For this review, take the finished solid that the model builds, in its own axes (mm). A direction names the side the tool comes from. Coordinates: 2 decimals unless noted, no trailing zeros. Loops run counter-clockwise (first coordinate to the right, second up) from the corner with the lowest first, then second, coordinate; pieces in that order, holes last. Notation, with made-up numbers: M -25,-8 L -13,-8 A24 ccw -13,19 Z; hole C 72,-5 d1. An arc over 180 degrees is marked long. Use one line per item in the form item = value.
```python
from build123d import *

# Parameters (mm, degrees)
SKETCH1_W           = 51.225
SKETCH1_H           = 33.05
BOSS_EXTRUDE1_DEPTH = 6.35
SKETCH8_R           = 1.25
CUT_EXTRUDE4_DEPTH  = 15
FILLET3_R           = 5.08
SKETCH10_R          = 3.35
SKETCH10_R_2        = 11.05
CUT_EXTRUDE5_DEPTH  = 4.7625
CHAMFER1_SIZE       = 0.25


with BuildPart() as part:
    # Sketch1 → Boss-Extrude1 (new body)
    with BuildSketch(Plane.XY):
        with Locations((-7.6125, 2.525)):
            Rectangle(SKETCH1_W, SKETCH1_H)
    extrude(amount=-BOSS_EXTRUDE1_DEPTH)

    # Sketch8 → Cut-Extrude4 (cut)
    with BuildSketch(Plane(origin=(0, 19.05, 0), x_dir=(1, 0, 0), z_dir=(0, 1, 0))):
        with Locations(Location((-29.725, 3.175, 0), (0, 0, 270))):
            Circle(SKETCH8_R)
        with Locations(Location((-14, 3.175, 0), (0, 0, 270))):
            Circle(SKETCH8_R)
        with Locations(Location((14.5, 3.175, 0), (0, 0, 270))):
            Circle(SKETCH8_R)
    extrude(amount=-CUT_EXTRUDE4_DEPTH, mode=Mode.SUBTRACT)

    # Fillet3
    fillet3_edges = [part.edges().sort_by_distance(p)[0] for p in [
        (18, -14, -3.175),
        (-33.225, -14, -3.175),
    ]]
    fillet(fillet3_edges, radius=FILLET3_R)

    # Sketch10 → Cut-Extrude5 (cut)
    with BuildSketch(Plane(origin=(0, 0, -6.35), x_dir=(-1, 0, 0), z_dir=(0, 0, -1))):
        with Locations((22.225, 0)):
            Circle(SKETCH10_R)
        Circle(SKETCH10_R_2)
    extrude(amount=-CUT_EXTRUDE5_DEPTH, mode=Mode.SUBTRACT)

    # Chamfer1
    chamfer1_edges = [part.edges().sort_by_distance(p)[0] for p in [
        (-29.725, 19.05, -4.425),
        (-14, 19.05, -4.425),
        (14.5, 19.05, -4.425),
    ]]
    chamfer(chamfer1_edges, length=CHAMFER1_SIZE)


solid = part.part
```
1. Tool access review of faces 1 (the face through (-31.78, -12.47, -3.22)), 2 (the face through (-28.486, 11.528, -3.338)), 3 (the face through (-22, 0, -1.587)): name each direction out of +Z, -Z, +X, -X, +Y, -Y from which nothing blocks a thin tool from reaching the whole face with its end or side.
Computed values:
face_1 = +Z, -Z, -X, -Y
face_2 = +Y
face_3 = -Z
2. Consider section D-D on z = -2.5. State how many separate pieces and enclosed holes the cut face has, plus the area to 3 significant figures.
Computed values:
separate_pieces = 1
enclosed_holes = 2
area = 1,170 mm2
3. Draft analysis for pull direction Z (two halves, no side actions). For faces 4 (the face through (2.395, -10.787, -4.002)), 5 (the face through (-14, 4.05, -3)), 6 (the face through (-8, 3, 0)), state which applies: +Z half, -Z half, draft (parallel to the pull), parting line (faces both ways), or undercut.
Computed values:
face_4 = draft
face_5 = undercut
face_6 = +Z half
4. Wall thickness on line 1 along Y through (x, z) = (0, -4.95); line 2 along X through (y, z) = (14, -3.5) (3 decimals); line 3 along X through (y, z) = (-6, -5.5) (3 decimals): over which ranges is each line inside the solid? List them lowest first. Write a range as from..to.
Computed values:
line_1 = -14..-11.05, 11.05..19.05
line_2 = -33.225..-30.932, -28.518..-15.207, -12.793..13.293, 15.707..18
line_3 = -33.225..-9.279, 9.279..18
5. Consider section B-B on x = -14. Write out the cut boundary in (y, z) (3 decimals), plus the area to 3 significant figures.
Computed values:
outline = M -14,-6.35 L 19.05,-6.35 L 19.05,-4.675 L 18.8,-4.425 L 4.05,-4.425 L 4.05,-1.925 L 18.8,-1.925 L 19.05,-1.675 L 19.05,0 L -14,0 Z
area = 172 mm2
6. For pin 1 Ø1.2 at (x, z) = (-30, -3) entering from +Y; pin 2 Ø1.5 at (x, z) = (14.5, -3.175) entering from -Y; pin 3 Ø6.5 at (x, y) = (4.5, 3) entering from -Z, all flat-tipped, find the tip position at first contact; note any pin that passes through.
Computed values:
pin_1 = 4.05
pin_2 = -13.93
pin_3 = -1.59
7. Consider section A-A on y = 13. Write out the cut boundary in (x, z) (3 decimals), plus the area to 3 significant figures.
Computed values:
outline = M -33.225,-6.35 L 18,-6.35 L 18,0 L -33.225,0 Z; hole C -29.725,-3.175 d2.5; hole C -14,-3.175 d2.5; hole C 14.5,-3.175 d2.5
area = 311 mm2
